Here's how the part is built. I have some questions about the finished solid (model axes, mm). Coordinates: 2 decimals unless noted, no trailing zeros. Write each loop counter-clockwise with the first axis right and the second up, starting at its lowest first coordinate (ties: lowest second). Pieces come first, ordered by that corner, then holes. Notation, with made-up numbers: (13, 50.25) -> (45, 50.25) arc R19 ccw to (45, 86.25) -> close; hole circle Ø6 at (-21, 63). An arc over 180 degrees is marked (long way). Use a Markdown table: item, result. Add a question column.
```python
from build123d import *

# Parameters (mm, degrees)
F0_R     = 20
F1_DEPTH = 0.7
F2_R     = 0.5
F3_DEPTH = 0.7


with BuildPart() as f1:
    # F0 (on Top) → F1 (new body)
    with BuildSketch(Plane.XY):
        Circle(F0_R)
    extrude(amount=F1_DEPTH)

    # F2 (on face) → F3 (cut)
    with BuildSketch(Plane.XY.offset(0.7)):
        with Locations((-12.942992, 0)):
            Circle(F2_R)
        with Locations((12.675214, 2.915508)):
            Circle(F2_R)
        with Locations((9.06239, -9.565156)):
            Circle(F2_R)
        Circle(F2_R)
        with Locations((-8.180633, 10.141156)):
            Circle(F2_R)
        with Locations((-6.045783, -10.386252)):
            Circle(F2_R)
        with Locations((6.106443, 12.111788)):
            Circle(F2_R)
    extrude(amount=-F3_DEPTH, mode=Mode.SUBTRACT)


solid = f1.part
```
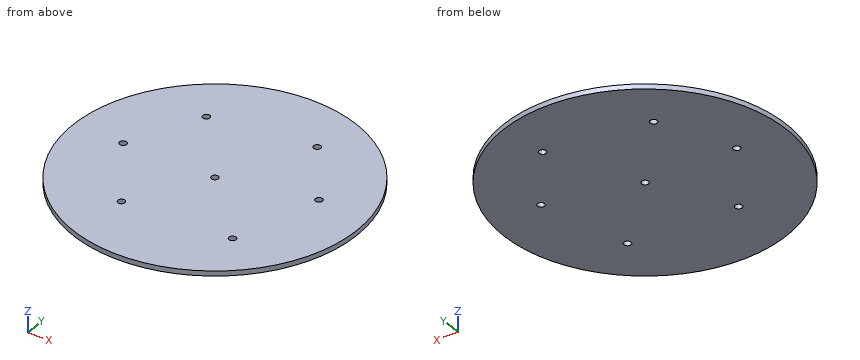
Q1. Suppose I cut it at A-A, the plane y = 0. Write out the boundary of the cut face in (x, z), and give its area (3 significant figures).
Q2. Suppose I cut it at C-C, the plane z = 0.55. Write out the boundary of the cut face in (x, y), and give its area (3 significant figures).
Q3. Suppose I cut it at B-B, the plane x = 0. Write out the boundary of the cut face in (y, z).
Q4. Please list where these lines run through material, in increasing order: line 1 (X direction, y = 10, z = 0.6); line 2 (Y direction, x = 16, z = 0.15); line 3 (X direction, y = -10.5, z = 0.45).
Q5. Suppose I cut it at D-D, the plane x = -16. Write out the boundary of the cut face in (y, z), and give its area (3 significant figures).
Answer key:
| question | item | result |
|---|---|---|
| 1 | outline | (-20, 0) -> (-13.44, 0) -> (-13.44, 0.7) -> (-20, 0.7) -> close; (-12.44, 0) -> (-0.5, 0) -> (-0.5, 0.7) -> (-12.44, 0.7) -> close; (0.5, 0) -> (20, 0) -> (20, 0.7) -> (0.5, 0.7) -> close |
| 1 | area | 26.6 mm^2 |
| 2 | outline | circle Ø40 at (0, 0); hole circle Ø1 at (-12.94, 0); hole circle Ø1 at (-8.18, 10.14); hole circle Ø1 at (-6.05, -10.39); hole circle Ø1 at (0, 0); hole circle Ø1 at (6.11, 12.11); hole circle Ø1 at (9.06, -9.57); hole circle Ø1 at (12.68, 2.92) |
| 2 | area | 1,250 mm^2 |
| 3 | outline | (-20, 0) -> (-0.5, 0) -> (-0.5, 0.7) -> (-20, 0.7) -> close; (0.5, 0) -> (20, 0) -> (20, 0.7) -> (0.5, 0.7) -> close |
| 4 | line 1 | x = -17.32 to -8.66, -7.7 to 17.32 |
| 4 | line 2 | y = -12 to 12 |
| 4 | line 3 | x = -17.02 to -6.53, -5.56 to 17.02 |
| 5 | outline | (-12, 0) -> (12, 0) -> (12, 0.7) -> (-12, 0.7) -> close |
| 5 | area | 16.8 mm^2 |
